Model file for the job. Use its own axes, mm. A direction names the side the tool comes from. Give positions to 0.01 mm unless a question says otherwise; leave off trailing zeros. Loops run counter-clockwise (first coordinate to the right, second up) from the corner with the lowest first, then second, coordinate; pieces in that order, holes last. Notation, with made-up numbers: M 28.5,16.25 L 35.5,16.25 A24 ccw 35.5,50.25 Z; hole C 63.5,14.25 d8. An arc over 180 degrees is marked long. Use CSV: the item, a comma, the result in double quotes. Start each with the question number.
(1) Flat gauge pins, fed straight in: P1, Ø4, axis at x = 22, y = 35.5, coming from the -Z side; P2, Ø0.6, axis at x = -10.5, z = -2, coming from the +Y side; P3, Ø5.5, axis at x = 0.5, y = 34.5, coming from the +Z side. Where does each tip first touch, or does it go through?
(2) Slice it at A-A on x = 0. List the corners of the cut face in (y, z).
(3) Tool access for faces 1 (the face through (-4, 35, -0.5)), 2 (the face through (-4, 37.295, -1)), 3 (the face through (32.7, 41.9, -24.1)), 4 (the face through (-4, 32.295, -2)): list every direction of +Z, -Z, +X, -X, +Y, -Y with a clear straight run to the whole face (end or side of a thin tool).
(4) Two-plate mould, pull along Y, no slides. Class faces 5 (the face through (-4, 41.295, -2)), 6 (the face through (34, 52.208, 0)), 7 (the face through (34, 40, -29.934)): pulls with the +Y half, pulls with the -Y half, needs draft (parallel to the pull), parting line crosses it, or undercut.
(5) Wall check: line 1 along X through (y, z) = (57.5, 1.5); line 2 along Z through (x, y) = (-1.5, 33.5); line 3 along Z through (x, y) = (52, 57.5). Give the ranges that are in metal, low to high. Write a range as from..to.
(6) Slice it at B-B on x = 34. List the corners of the cut face in (y, z), and give its area (3 significant figures).
(7) Slice it at C-C on y = 56. List the corners of the cut face in (x, z).
Autodesk Inventor part; units mm, degrees
ref_plane "XZ Plane" through (0, 0, 0) normal (0, 1, 0) x (-1, 0, 0)
ref_plane "XY Plane" through (0, 0, 0) normal (0, 0, 1) x (1, 0, 0)
ref_plane "Work Plane2" through (-80, 0, -3) normal (0, 0, -1) x (-1, 0, 0)
sketch "Sketch1" plane through (0, 0, 0) normal (0, 0, 1) x (1, 0, 0)
  line L0 (34, 31.2954) -> (15.654, 31.2954)
  line L1 (15.654, 31.2954) -> (15.654, 48.2362)
  line L2 (15.654, 48.2362) -> (1.0463, 64.8622)
  line L3 (1.0463, 64.8622) -> (1.0463, 69.6686)
  line L4 (1.0463, 69.6686) -> (2.3392, 69.6686)
  line L5 (2.3392, 69.6686) -> (17.6799, 52.2084)
  line L6 (17.6799, 52.2084) -> (34, 52.2084)
  line L7 (52, 820) -> (16, 820)
  line L8 (34, 820) -> (34, 0)
  point P0 (0, 0)
revolve "Revolution1" add sketch "Sketch1" angle 360 about axis through (34, 820, 0) along (0, -1, 0)
ref_plane "Work Plane1" through (15.654, 39.7658, 0) normal (1, 0, 0) x (0, 1, 0)
sketch "Sketch2" plane through (15.654, 39.7658, 0) normal (1, 0, 0) x (0, 1, 0)
  line L0 (-8.4704, -18.346) -> (-8.4704, 18.346) construction
  line L1 (-2.4704, -2.5) -> (-7.4704, -2.5)
  line L2 (-7.4704, -2.5) -> (-7.4704, -0.5)
  line L3 (-7.4704, -0.5) -> (-2.4704, -0.5)
  line L4 (-2.4704, -0.5) -> (-2.4704, -2.5)
  line L5 (6.5296, -2.5) -> (1.5296, -2.5)
  line L6 (1.5296, -2.5) -> (1.5296, -0.5)
  line L7 (1.5296, -0.5) -> (6.5296, -0.5)
  line L8 (6.5296, -0.5) -> (6.5296, -2.5)
  line L9 (6.5296, -2.5) -> (1.5296, -0.5) construction
  line L10 (6.5296, -0.5) -> (1.5296, -2.5) construction
  line L11 (-7.4704, -0.5) -> (-2.4704, -2.5) construction
  line L12 (-7.4704, -2.5) -> (-2.4704, -0.5) construction
  line L13 (-39.7658, 0) -> (810.2342, 0)
  dimension "d1" = 5
  dimension "d2" = 2
  dimension "d3" = 1
  dimension "d4" = 4
  dimension "d10" = 0.5
extrude "Extrusion1" add sketch "Sketch2" along normal blind 2.0625 and the other way blind 38.3375
ref_plane "Work Plane3" through (34, 39.7658, -18.346) normal (0, 0, -1) x (-1, 0, 0)
ref_plane "Work Plane2" through (-80, 0, -3) normal (0, 0, -1) x (-1, 0, 0)
sketch "Sketch3" plane through (34, 39.7658, -18.346) normal (0, 0, -1) x (-1, 0, 0)
  circle A0 centre (0, 0) radius 2.5
  circle A1 centre (0, 779.9029) radius 2.5
  point P0 (34, -39.7658)
extrude "Extrusion2" add sketch "Sketch3" along normal blind 11.5875 and the other way blind 5.7935 contours A0
properties part number "BallReciever"
Reply:
1,P1,"stops at z = -15.38"
1,P2,"stops at y = 46.3"
1,P3,"stops at z = -0.5"
2,outline,"M 32.3,-2.5 L 37.3,-2.5 L 37.3,-0.5 L 32.3,-0.5 Z; M 41.3,-2.5 L 46.3,-2.5 L 46.3,-0.5 L 41.3,-0.5 Z"
3,face 1,"+Z, -X, -Y"
3,face 2,"+Z, -Z, -X"
3,face 3,"-Z"
3,face 4,"+Z, -Z, -X, -Y"
4,face 5,"undercut"
4,face 6,"pulls with the +Y half"
4,face 7,"needs draft"
5,line 1,"x = 7.56..13.08, 54.92..60.44"
5,line 2,"z = -2.5..-0.5"
5,line 3,"z = -19.43..-10.76, 10.76..19.43"
6,outline,"M 31.3,-18.35 L 37.27,-18.35 L 37.27,-29.93 L 42.27,-29.93 L 42.27,-18.35 L 48.24,-18.35 L 64.86,-32.95 L 69.67,-32.95 L 69.67,-31.66 L 52.21,-16.32 L 52.21,16.32 L 69.67,31.66 L 69.67,32.95 L 64.86,32.95 L 48.24,18.35 L 31.3,18.35 Z"
6,area,"1,010 mm^2"
7,outline,"C 34,0 d50.33; hole C 34,0 d39.3"
